Could you check a few things on this drawing? It's one solid part, dimensions in mm from its lowest x, y, z. Coordinates: 2 decimals unless noted, no trailing zeros. Order: outer loops, then holes, each group sorted by start corner. A loop starts at its lowest first (then second) coordinate and runs counter-clockwise, first axis right, second up. Notation, with made-up numbers: (-18, -30) -> (18, -30) arc R24 cw to (18, -3) -> close; hole circle Ø11 at (-16, 55). An arc over 180 degrees is marked (long way). Use a Markdown table: item, result. Add a question column.
1. Suppose I cut it at D-D, the plane x = 35.5. List the corners of the cut face in (y, z) for me (1 decimal).
2. If I drill on line 1 along X through (y, z) = (7.75, 14) (1 decimal); line 2 along X through (y, z) = (8.25, 11.5) (1 decimal); line 3 along X through (y, z) = (2, 4) (1 decimal), over which ranges is the centre line in solid material (lowest first)? Write a range as from..to.
3. We'd pull the mould along X, two halves only. Please class the marked faces 1, 2, 3 and 4: pulls with the +X half, pulls with the -X half, needs draft (parallel to the pull), parting line crosses it, or undercut.
4. Suppose I cut it at B-B, the plane y = 10. List the corners of the cut face in (x, z) for me (1 decimal).
5. Suppose I cut it at A-A, the plane z = 13.75. State how many separate pieces and enclosed holes the cut face has, then the cut area to 3 significant figures.
6. For pin 1 Ø6 at (x, z) = (21, 11) entering from +Y; pin 2 Ø5 at (x, y) = (24.5, 3) entering from +Z (1 decimal), each with a flat end and sliding along its axis, tell me the tip position at first contact or that it passes through.
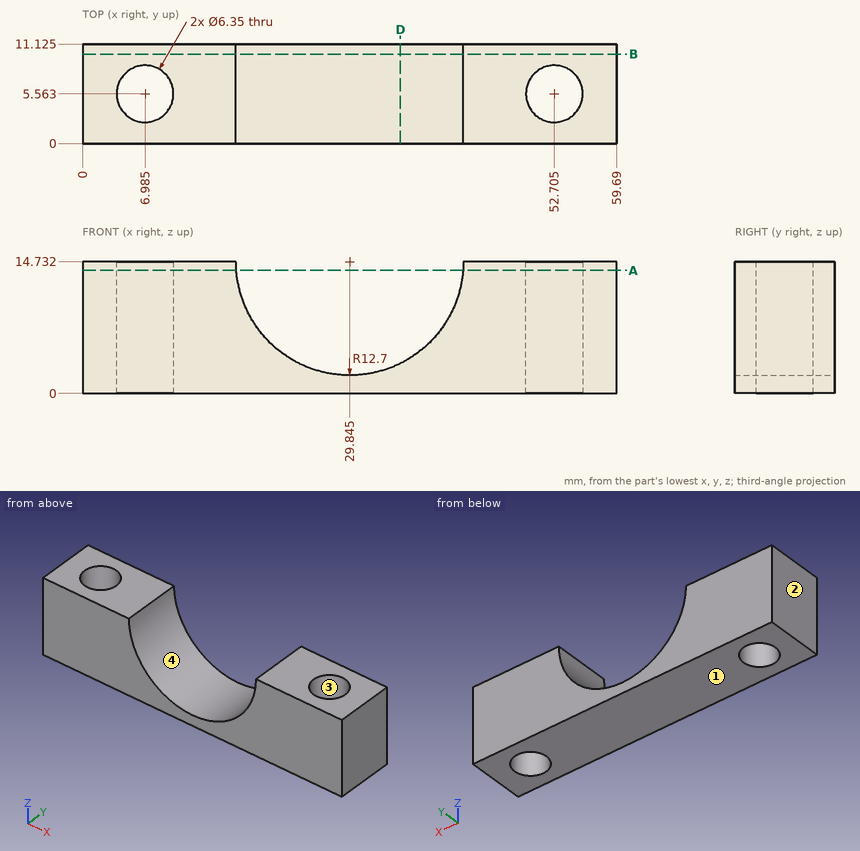
Worked out:
| question | item | result |
|---|---|---|
| 1 | outline | (0, 0) -> (11.1, 0) -> (11.1, 3.4) -> (0, 3.4) -> close |
| 2 | line 1 | x = 0..4.7, 9.3..17.2, 42.5..50.4, 55..59.7 |
| 2 | line 2 | x = 0..5.3, 8.7..17.6, 42.1..51, 54.4..59.7 |
| 2 | line 3 | x = 0..23.1, 36.6..59.7 |
| 3 | face 1 | needs draft |
| 3 | face 2 | pulls with the -X half |
| 3 | face 3 | undercut |
| 3 | face 4 | undercut |
| 4 | outline | (0, 0) -> (59.7, 0) -> (59.7, 14.7) -> (42.5, 14.7) arc R12.7 cw to (17.1, 14.7) -> (0, 14.7) -> close |
| 5 | separate pieces | 2 |
| 5 | enclosed holes | 2 |
| 5 | area | 319 mm² |
| 6 | pin 1 | passes through |
| 6 | pin 2 | stops at z = 4.7 |
